Work out the finished part from the listing and answer in its coordinate system (mm). A direction names the side the tool comes from. Round coordinates to 2 decimals unless told otherwise and drop trailing zeros. Loops run counter-clockwise (first coordinate to the right, second up) from the corner with the lowest first, then second, coordinate; pieces in that order, holes last. Notation, with made-up numbers: (76, 63) -> (133, 63) arc R33 ccw to (133, 101) -> close; hole circle Ø1 at (87.25, 9). An arc over 180 degrees is marked (long way). Use one line per item in the form item = value.
```python
from build123d import *

# Parameters (mm, degrees)
SKETCH1_W             = 3.175
SKETCH1_H             = 12.7
CHAMFER1_SIZE         = 0.9525
BODY_MOVE_COPY1_ANGLE = 180
SKETCH4_W             = 7.9375
SKETCH4_H             = 15.875


with BuildPart() as part:
    # Sketch1 → Revolve1 (revolve)
    with BuildSketch(Plane.XY, mode=Mode.PRIVATE) as revolve1_sk:
        with Locations((1.5875, 14.2875)):
            Rectangle(SKETCH1_W, SKETCH1_H)
    revolve(revolve1_sk.sketch.rotate(Axis((0, 7.9375, 0), (0, 1, 0)), 90), axis=Axis((0, 7.9375, 0), (0, 1, 0)))

    # Chamfer1
    chamfer1_edges = [part.edges().sort_by_distance(p)[0] for p in [
        (0, 20.6375, 3.175),
    ]]
    chamfer(chamfer1_edges, length=CHAMFER1_SIZE)


with BuildPart() as body_2:
    # Body-Move_Copy1: copy of part
    add(part.part.rotate(Axis((0, 0, 0), (1, 0, 0)), BODY_MOVE_COPY1_ANGLE))


with BuildPart() as part_1:
    add(part.part)

    add(body_2.part)  # Revolve2 merges body 2
    # Sketch4 → Revolve2 (revolve)
    with BuildSketch(Plane.XY):
        with Locations((3.96875, 0)):
            Rectangle(SKETCH4_W, SKETCH4_H)
    revolve(axis=Axis((0, -7.9375, 0), (0, 1, 0)))


solid = part_1.part
```
(1) Given P1, Ø3, axis at y = -3, z = -4.5, coming from the -X side; P2, Ø8, axis at x = 0, z = 3, coming from the -Y side; P3, Ø6, axis at y = 3, z = 3.5, coming from the +X side; P4, Ø3, axis at x = -5.5, y = 2.5, coming from the +Z side, each flat-ended and moving along its own axis, determine where each tip first touches the part or whether it passes through.
Completed:
P1 = -7.35
P2 = -20.64
P3 = 7.92
P4 = 6.86
(2) Consider L1, parallel to Y at x = 4, z = 5.75; L2, parallel to Z at x = 0.25, y = 2; L3, parallel to Z at x = 4.25, y = -3.5. Determine where each line is inside the solid, lowest interval first.
Completed:
L1 = -7.94 to 7.94
L2 = -7.93 to 7.93
L3 = -6.7 to 6.7
(3) Find section B-B, the plane z = 0. Write down the section's boundary in (x, y) (1 decimal).
Completed:
outline = (-7.9, -7.9) -> (-3.2, -7.9) -> (-3.2, -19.7) -> (-2.2, -20.6) -> (2.2, -20.6) -> (3.2, -19.7) -> (3.2, -7.9) -> (7.9, -7.9) -> (7.9, 7.9) -> (3.2, 7.9) -> (3.2, 19.7) -> (2.2, 20.6) -> (-2.2, 20.6) -> (-3.2, 19.7) -> (-3.2, 7.9) -> (-7.9, 7.9) -> close
(4) Find section C-C, the plane y = -3. Write down the section's boundary in (x, z) (1 decimal).
Completed:
outline = circle Ø15.9 at (0, 0)
(5) Find section D-D, the plane y = -13.5. Write down the section's boundary in (x, z) (3 decimals).
Completed:
outline = circle Ø6.35 at (0, 0)
(6) Find section A-A, the plane x = 0. Write down the section's boundary in (y, z) (1 decimal).
Completed:
outline = (-20.6, -2.2) -> (-19.7, -3.2) -> (-7.9, -3.2) -> (-7.9, -7.9) -> (7.9, -7.9) -> (7.9, -3.2) -> (19.7, -3.2) -> (20.6, -2.2) -> (20.6, 2.2) -> (19.7, 3.2) -> (7.9, 3.2) -> (7.9, 7.9) -> (-7.9, 7.9) -> (-7.9, 3.2) -> (-19.7, 3.2) -> (-20.6, 2.2) -> close
(7) For faces 1 (the flat face through (-3.4, 7.938, -0.1)), 2 (the flat face through (0, -20.638, 0)), 3 (the cylindrical face through (2.8, -13.9, 1.5)), determine the directions among +Z, -Z, +X, -X, +Y, -Y from which every point of the face is accessible in a straight line to the end or side of a thin tool.
Completed:
face_1 = +Y
face_2 = +Z, -Z, +X, -X, -Y
face_3 = -Y
